Check sheet for the modelled part. Datum: model origin and axes. Units: mm. A direction names the side the tool comes from. Round coordinates to 2 decimals unless told otherwise and drop trailing zeros. Loops run counter-clockwise (first coordinate to the right, second up) from the corner with the lowest first, then second, coordinate; pieces in that order, holes last. Notation, with made-up numbers: (36.25, 63) - (62.25, 63) arc R32 cw to (62.25, 94) - close; hole circle Ø10 at (41, 8). An arc over 180 degrees is marked (long way). Return JSON: item names as keys, results as strings.
from build123d import *

# Parameters (mm, degrees)
BOSS_EXTRUDE1_DEPTH = 11
CUT_EXTRUDE1_DEPTH  = 22
CUT_EXTRUDE2_START  = 12
CUT_EXTRUDE2_DEPTH  = 1
SKETCH3_R           = 4
SKETCH3_R_2         = 1.75
CUT_EXTRUDE3_DEPTH  = 41
CUT_EXTRUDE6_START  = 31
SKETCH3_4_R         = 3.5
SKETCH3_4_R_2       = 1.75
CUT_EXTRUDE6_DEPTH  = 1
FILLET1_R           = 10
CUT_EXTRUDE7_START  = 28
SKETCH3_5_R         = 4
CUT_EXTRUDE7_DEPTH  = 1.5
FILLET2_R           = 0.5
FILLET3_R           = 1


with BuildPart() as part:
    # Sketch1 → Boss-Extrude1 (new body, symmetric)
    with BuildSketch(Plane.XY):
        with BuildLine():
            Line((-14, 12), (16, 12))
            Line((16, 12), (18, 12))
            Line((18, 12), (28, 22))
            Line((28, 22), (28, 24))
            Line((28, 24), (28, 49))
            Line((28, 49), (28, 52))
            Line((28, 52), (31, 52))
            Line((31, 52), (31, 49))
            Line((31, 49), (31, 27))
            Line((31, 27), (31, 22.757359313))
            Line((31, 22.757359313), (31, 21))
            ThreePointArc((31, 21), (27.485281374, 12.514718626), (19, 9))
            Line((19, 9), (17.242640687, 9))
            Line((17.242640687, 9), (14, 9))
            Line((14, 9), (-14, 9))
            Line((-14, 9), (-19, 9))
            Line((-19, 9), (-19, 12))
            Line((-19, 12), (-14, 12))
        make_face()
    extrude(amount=BOSS_EXTRUDE1_DEPTH, both=True)

    # Sketch2 → Cut-Extrude1 (cut)
    with BuildSketch(Plane(origin=(0, 0, 0), x_dir=(1, 0, 0), z_dir=(0, 1, 0))):
        with BuildLine():
            Line((-15, 1.25), (15, 1.25))
            ThreePointArc((15, 1.25), (16.25, 0), (15, -1.25))
            Line((15, -1.25), (-15, -1.25))
            ThreePointArc((-15, -1.25), (-16.25, 0), (-15, 1.25))
        make_face()
        with BuildLine():
            Line((-9, 7.25), (9, 7.25))
            ThreePointArc((9, 7.25), (10.25, 6), (9, 4.75))
            Line((9, 4.75), (-9, 4.75))
            ThreePointArc((-9, 4.75), (-10.25, 6), (-9, 7.25))
        make_face()
        with BuildLine():
            Line((-9, -7.25), (9, -7.25))
            ThreePointArc((9, -7.25), (10.25, -6), (9, -4.75))
            Line((9, -4.75), (-9, -4.75))
            ThreePointArc((-9, -4.75), (-10.25, -6), (-9, -7.25))
        make_face()
    extrude(amount=CUT_EXTRUDE1_DEPTH, mode=Mode.SUBTRACT)

    # Sketch2_4 → Cut-Extrude2 (cut)
    with BuildSketch(Plane(origin=(0, 0, 0), x_dir=(1, 0, 0), z_dir=(0, 1, 0)).offset(CUT_EXTRUDE2_START)):
        with BuildLine():
            Line((-9, 8.25), (9, 8.25))
            ThreePointArc((9, 8.25), (11.25, 6), (9, 3.75))
            Line((9, 3.75), (-9, 3.75))
            ThreePointArc((-9, 3.75), (-11.25, 6), (-9, 8.25))
        make_face()
        with BuildLine():
            Line((-15, 2.25), (15, 2.25))
            ThreePointArc((15, 2.25), (17.25, 0), (15, -2.25))
            Line((15, -2.25), (-15, -2.25))
            ThreePointArc((-15, -2.25), (-17.25, 0), (-15, 2.25))
        make_face()
        with BuildLine():
            Line((-9, -8.25), (9, -8.25))
            ThreePointArc((9, -8.25), (11.25, -6), (9, -3.75))
            Line((9, -3.75), (-9, -3.75))
            ThreePointArc((-9, -3.75), (-11.25, -6), (-9, -8.25))
        make_face()
    extrude(amount=-CUT_EXTRUDE2_DEPTH, mode=Mode.SUBTRACT)

    # Sketch3 → Cut-Extrude3 (cut)
    with BuildSketch(Plane(origin=(0, 0, 0), x_dir=(0, 0, -1), z_dir=(1, 0, 0))):
        with BuildLine():
            ThreePointArc((14, 38), (0, 52), (-14, 38))
            Line((-14, 38), (-18.083986214, 38))
            Line((-18.083986214, 38), (-18.083986214, 55.660635954))
            Line((-18.083986214, 55.660635954), (16.65758444, 55.660635954))
            Line((16.65758444, 55.660635954), (16.65758444, 38))
            Line((16.65758444, 38), (14, 38))
        make_face()
        with Locations((11.00722034, 26.99277966)):
            Circle(SKETCH3_R)
        with Locations(Location((-8, 38, 0), (0, 0, 180))):  # turned: the seam where the file's is
            Circle(SKETCH3_R_2)
        with Locations(Location((0, 28.5, 0), (0, 0, 180))):  # turned: the seam where the file's is
            Circle(SKETCH3_R_2)
        with Locations(Location((8, 38, 0), (0, 0, 180))):  # turned: the seam where the file's is
            Circle(SKETCH3_R_2)
        with Locations(Location((0, 47.5, 0), (0, 0, 180))):  # turned: the seam where the file's is
            Circle(SKETCH3_R_2)
    extrude(amount=CUT_EXTRUDE3_DEPTH, mode=Mode.SUBTRACT)

    # Sketch3_4 → Cut-Extrude6 (cut)
    with BuildSketch(Plane(origin=(0, 0, 0), x_dir=(0, 0, -1), z_dir=(1, 0, 0)).offset(CUT_EXTRUDE6_START)):
        with Locations(Location((0, 28.5, 0), (0, 0, 180))):  # turned: the seam where the file's is
            Circle(SKETCH3_4_R)
        with Locations(Location((0, 28.5, 0), (0, 0, 180))):  # turned: the seam where the file's is
            Circle(SKETCH3_4_R_2, mode=Mode.SUBTRACT)
        with Locations((-8, 38)):
            Circle(SKETCH3_4_R)
        with Locations(Location((-8, 38, 0), (0, 0, 180))):  # turned: the seam where the file's is
            Circle(SKETCH3_4_R_2, mode=Mode.SUBTRACT)
        with Locations(Location((0, 47.5, 0), (0, 0, 180))):  # turned: the seam where the file's is
            Circle(SKETCH3_4_R)
        with Locations(Location((0, 47.5, 0), (0, 0, 180))):  # turned: the seam where the file's is
            Circle(SKETCH3_4_R_2, mode=Mode.SUBTRACT)
        with Locations((8, 38)):
            Circle(SKETCH3_4_R)
        with Locations(Location((8, 38, 0), (0, 0, 180))):  # turned: the seam where the file's is
            Circle(SKETCH3_4_R_2, mode=Mode.SUBTRACT)
    extrude(amount=-CUT_EXTRUDE6_DEPTH, mode=Mode.SUBTRACT)

    # Fillet1
    fillet1_edges = [part.edges().sort_by_distance(p)[0] for p in [
        (-19, 10.5, -11),
        (-19, 10.5, 11),
    ]]
    fillet(fillet1_edges, radius=FILLET1_R)

    # Sketch3_5 → Cut-Extrude7 (cut)
    with BuildSketch(Plane(origin=(0, 0, 0), x_dir=(0, 0, -1), z_dir=(1, 0, 0)).offset(CUT_EXTRUDE7_START)):
        with Locations((0, 38)):
            Circle(SKETCH3_5_R)
    extrude(amount=CUT_EXTRUDE7_DEPTH, mode=Mode.SUBTRACT)

    # Fillet2
    fillet2_edges = [part.edges().sort_by_distance(p)[0] for p in [
        (29.5, 22.992786177, -11),
        (29.5, 30.992773143, -11),
        (28, 26.99277966, -7.00722034),
        (31, 26.99277966, -7.00722034),
        (28, 38, 4),
    ]]
    fillet(fillet2_edges, radius=FILLET2_R)

    # Fillet3
    fillet3_edges = [part.edges().sort_by_distance(p)[0] for p in [
        (18, 12, 0),
        (28, 22, 0),
    ]]
    fillet(fillet3_edges, radius=FILLET3_R)


solid = part.part
Q1. Sectioned sample at D-D (x = 21). Enter the section's corners in (y, z).
Answer key:
{"outline": "(9.17, -11) - (15, -11) - (15, 11) - (9.17, 11) - close"}
Q2. Draft check along Y on faces 4 (the face through (0, 9, 3)), 5 (the face through (30.5, 37.9, 4.5)), 6 (the face through (31, 37, 0)). Enter one of: released by +Y, released by -Y, zero draft, split by the parting line, or undercut.
Answer key:
{"face 4": "released by -Y", "face 5": "undercut", "face 6": "zero draft"}
Q3. Sectioned sample at B-B (y = 47.5). Enter the section's corners in (x, z), plus the area to 3 significant figures.
Answer key:
{"outline": "(28, -10.28) - (31, -10.28) - (31, -3.5) - (30, -3.5) - (30, -1.75) - (28, -1.75) - close; (28, 1.75) - (30, 1.75) - (30, 3.5) - (31, 3.5) - (31, 10.28) - (28, 10.28) - close", "area": "47.7 mm²"}
Q4. Depth check by flat-ended pin: P1, Ø10.5, axis at y = 38, z = 0, coming from the -X side; P2, Ø6.5, axis at y = 38, z = -8, coming from the +X side; P3, Ø3.5, axis at x = 1.5, z = -6, coming from the +Y side; P4, Ø10, axis at x = 20, y = 40, coming from the +Z side. Enter the tip coordinate at first touch or a pass-through.
Answer key:
{"P1": "stops at x = 28", "P2": "stops at x = 30", "P3": "stops at y = 11", "P4": "passes through"}
Q5. Sectioned sample at A-A (x = -1.5). Enter the section's corners in (y, z).
Answer key:
{"outline": "(9, -11) - (12, -11) - (12, -8.25) - (11, -8.25) - (11, -7.25) - (9, -7.25) - close; (9, -4.75) - (11, -4.75) - (11, -3.75) - (12, -3.75) - (12, -2.25) - (11, -2.25) - (11, -1.25) - (9, -1.25) - close; (9, 1.25) - (11, 1.25) - (11, 2.25) - (12, 2.25) - (12, 3.75) - (11, 3.75) - (11, 4.75) - (9, 4.75) - close; (9, 7.25) - (11, 7.25) - (11, 8.25) - (12, 8.25) - (12, 11) - (9, 11) - close"}
Q6. Sectioned sample at C-C (z = 0). State how many separate pieces and enclosed holes the cut face has, plus the area to 3 significant figures.
Answer key:
{"separate pieces": "4", "enclosed holes": "0", "area": "150 mm²"}
Q7. Scan lines: probe 1 along Y at (x, z) = (28.55, 0); probe 2 along Y at (x, z) = (28.9, 0); probe 3 along Y at (x, z) = (7.5, 9.25). Record each from-to range of solid material in increasing order. Write a range as [from, to].
Answer key:
{"probe 1": "y = [13.73, 26.75], [30.25, 34], [42, 45.75], [49.25, 52]", "probe 2": "y = [14.22, 26.75], [30.25, 34], [42, 45.75], [49.25, 52]", "probe 3": "y = [9, 12]"}
Q8. Tool access check on faces 1 (the face through (28.993, 41.966, 0.521)), 2 (the face through (30, 48, -2)), 3 (the face through (17.25, 11.51, -0.05)). Record the directions out of +Z, -Z, +X, -X, +Y, -Y that give a thin tool (end or side, any length) a straight path to the whole face; none if there is none.
Answer key:
{"face 1": "-X", "face 2": "+X", "face 3": "+Y"}
